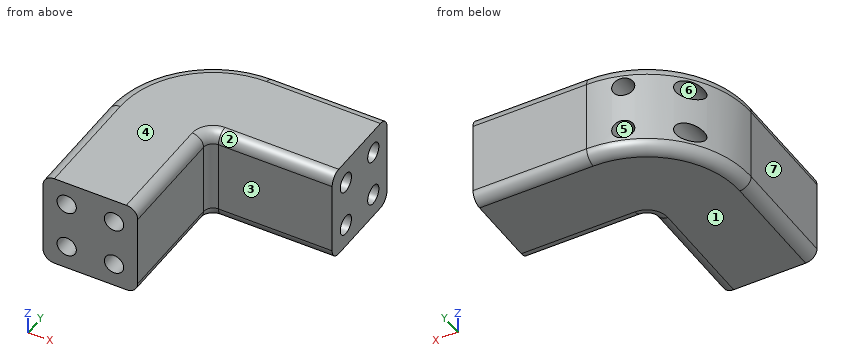
from build123d import *

# Parameters (mm, degrees)
SKETCH_3_R          = 2.55
CUT_EXTRUDE_1_DEPTH = 30
SKETCH_5_R          = 2.55
CUT_EXTRUDE_2_DEPTH = 75.077662045


with BuildPart() as part:
    # 扫描1: sweep along a path in 草图2
    with BuildLine(Plane.XY) as sweep_1_path:
        Line((0, 0), (0, 30))
        ThreePointArc((0, 30), (4.393398282, 40.606601718), (15, 45))
        Line((15, 45), (45, 45))
    # 草图1 → 扫描1 (sweep)
    with BuildSketch(Plane(origin=(0, 0, 0), x_dir=(1, 0, 0), z_dir=(0, 1, 0))):
        with BuildLine():
            Line((-9.5, 12.5), (9.5, 12.5))
            ThreePointArc((9.5, 12.5), (11.621320344, 11.621320344), (12.5, 9.5))
            Line((12.5, 9.5), (12.5, -9.5))
            ThreePointArc((12.5, -9.5), (11.621320344, -11.621320344), (9.5, -12.5))
            Line((9.5, -12.5), (-9.5, -12.5))
            ThreePointArc((-9.5, -12.5), (-11.621320344, -11.621320344), (-12.5, -9.5))
            Line((-12.5, -9.5), (-12.5, 9.5))
            ThreePointArc((-12.5, 9.5), (-11.621320344, 11.621320344), (-9.5, 12.5))
        make_face()
    sweep(path=sweep_1_path.line)

    # 草图3 → 切除-拉伸1 (cut)
    with BuildSketch(Plane(origin=(45, 0, 0), x_dir=(0, 0, -1), z_dir=(1, 0, 0))):
        with Locations(Location((6.25, 51.25, 0), (0, 0, 90))):
            Circle(SKETCH_3_R)
        with Locations(Location((6.25, 38.75, 0), (0, 0, 90))):
            Circle(SKETCH_3_R)
        with Locations(Location((-6.25, 38.75, 0), (0, 0, 90))):
            Circle(SKETCH_3_R)
        with Locations(Location((-6.25, 51.25, 0), (0, 0, 90))):
            Circle(SKETCH_3_R)
    extrude(amount=-CUT_EXTRUDE_1_DEPTH, mode=Mode.SUBTRACT)

    # 草图5 → 切除-拉伸2 (cut, through all)
    with BuildSketch(Plane.XZ):
        with Locations(Location((-6.25, 6.25, 0), (0, 0, 270))):
            Circle(SKETCH_5_R)
        with Locations(Location((6.25, 6.25, 0), (0, 0, 270))):
            Circle(SKETCH_5_R)
        with Locations(Location((-6.25, -6.25, 0), (0, 0, 270))):
            Circle(SKETCH_5_R)
        with Locations(Location((6.25, -6.25, 0), (0, 0, 270))):
            Circle(SKETCH_5_R)
    extrude(amount=-CUT_EXTRUDE_2_DEPTH, mode=Mode.SUBTRACT)


solid = part.part
Part model, mm, in its own coordinate system. Face numbers are marked on the shaded views. A direction names the side the tool comes from. Round coordinates to 2 decimals unless told otherwise and drop trailing zeros. Write each loop counter-clockwise with the first axis right and the second up, starting at its lowest first coordinate (ties: lowest second). Pieces come first, ordered by that corner, then holes. Notation, with made-up numbers: M -2,54.25 L 40,54.25 A16 ccw 40,81.25 Z; hole C 78.5,57 d6. An arc over 180 degrees is marked long. Return JSON: item names as keys, results as strings. Group by question number.
(1) Two-plate mould, pull along X, no slides. Class the marked faces 4, 5, 6 and 7: +X half, -X half, draft (parallel to the pull), parting line (faces both ways), or undercut.
(2) Saw through at A-A on x = 18. Write the cut outline in (y, z).
(3) Saw through at C-C on z = -6.25. Write the cut outline in (x, y), then the cut area to 3 significant figures.
(4) Drill centre lines: probe 1 along Z at (x, y) = (6.25, 33); probe 2 along X at (y, z) = (28.5, 4.5). Where is each one in solid material? Low to high.
(5) Pin check, flat tips, straight feed: pin 1 Ø3 at (y, z) = (38.75, -6.25) entering from +X; pin 2 Ø3 at (y, z) = (51.25, 6.25) entering from -X; pin 3 Ø5.5 at (y, z) = (8, -1) entering from +X. Stop position of each tip, or through.
(6) Saw through at D-D on z = -2. Write the cut outline in (x, y).
(7) Which spindle directions (+Z, -Z, +X, -X, +Y, -Y) get a long thin tool onto all of the face, cutting with end or side? Do the marked faces 1, 2 and 3. Say none if no direction does.
(8) Saw through at B-B on y = 13. Write the cut outline in (x, z).
Returned:
{
 "1": {"face 4": "draft", "face 5": "undercut", "face 6": "undercut", "face 7": "-X half"},
 "2": {"outline": "M 32.5,-9.5 A3 ccw 35.5,-12.5 L 54.5,-12.5 A3 ccw 57.5,-9.5 L 57.5,9.5 A3 ccw 54.5,12.5 L 35.5,12.5 A3 ccw 32.5,9.5 Z; hole C 38.75,-6.25 d5.1; hole C 38.75,6.25 d5.1; hole C 51.25,-6.25 d5.1; hole C 51.25,6.25 d5.1"},
 "3": {"outline": "M -12.5,0 L -8.8,0 L -8.8,43.78 A27.5 ccw -12.5,30 Z; M -3.7,0 L 3.7,0 L 3.7,55.07 A27.5 ccw -3.7,50.16 Z; M 8.8,0 L 12.5,0 L 12.5,30 A2.5 cw 15,32.5 L 45,32.5 L 45,36.2 L 15,36.2 L 15,41.3 L 45,41.3 L 45,48.7 L 15,48.7 L 15,53.8 L 45,53.8 L 45,57.5 L 15,57.5 A27.5 ccw 8.8,56.79 Z", "area": "1,260 mm²"},
 "4": {"probe 1": "-12.5 to -8.8, -3.7 to 3.7, 8.8 to 12.5", "probe 2": "-12.5 to -8.1, -4.4 to 4.4, 8.1 to 12.5"},
 "5": {"pin 1": "x = 15", "pin 2": "x = -3.85", "pin 3": "x = 12.5"},
 "6": {"outline": "M -12.5,0 L 12.5,0 L 12.5,30 A2.5 cw 15,32.5 L 45,32.5 L 45,57.5 L 15,57.5 A27.5 ccw -12.5,30 Z"},
 "7": {"face 1": "-Z, +X, -X, +Y, -Y", "face 2": "+Z, +X, -Y", "face 3": "+Z, -Z, +X, -Y"},
 "8": {"outline": "M -12.5,-9.5 A3 ccw -9.5,-12.5 L 9.5,-12.5 A3 ccw 12.5,-9.5 L 12.5,9.5 A3 ccw 9.5,12.5 L -9.5,12.5 A3 ccw -12.5,9.5 Z; hole C -6.25,-6.25 d5.1; hole C -6.25,6.25 d5.1; hole C 6.25,-6.25 d5.1; hole C 6.25,6.25 d5.1"}
}
